```python
from build123d import *

# Parameters (mm, degrees)
SKETCH1_W           = 111
SKETCH1_H           = 170.0625
BOSS_EXTRUDE1_DEPTH = 3
SKETCH2_W           = 111
SKETCH2_H           = 170.0625
SKETCH2_W_2         = 105
SKETCH2_H_2         = 164.0625
BOSS_EXTRUDE2_DEPTH = 131.25
SKETCH3_R           = 47
CUT_EXTRUDE1_DEPTH  = 3


with BuildPart() as part:
    # Sketch1 → Boss-Extrude1 (new body)
    with BuildSketch(Plane(origin=(0, 0, 0), x_dir=(1, 0, 0), z_dir=(0, 1, 0))):
        with Locations((55.5, -85.03125)):
            Rectangle(SKETCH1_W, SKETCH1_H)
    extrude(amount=BOSS_EXTRUDE1_DEPTH)

    # Sketch2 → Boss-Extrude2 (add)
    with BuildSketch(Plane(origin=(0, 3, 0), x_dir=(1, 0, 0), z_dir=(0, 1, 0))):
        with Locations((55.5, -85.03125)):
            Rectangle(SKETCH2_W, SKETCH2_H)
        with Locations((55.5, -85.03125)):
            Rectangle(SKETCH2_W_2, SKETCH2_H_2, mode=Mode.SUBTRACT)
    extrude(amount=BOSS_EXTRUDE2_DEPTH)

    # Sketch3 → Cut-Extrude1 (cut)
    with BuildSketch(Plane(origin=(0, 0, 0), x_dir=(-1, 0, 0), z_dir=(0, -1, 0))):
        with Locations(Location((-55.5, -85.03125, 0), (0, 0, 90))):
            Circle(SKETCH3_R)
    extrude(amount=-CUT_EXTRUDE1_DEPTH, mode=Mode.SUBTRACT)


solid = part.part
```
Read the model definition and answer for the solid it produces. Units are mm, in the model's axes. A direction names the side the tool comes from. Round coordinates to 2 decimals unless told otherwise and drop trailing zeros. Write each loop counter-clockwise with the first axis right and the second up, starting at its lowest first coordinate (ties: lowest second). Pieces come first, ordered by that corner, then holes. Notation, with made-up numbers: (-11, 5) - (26, 5) arc R18 ccw to (26, 9) - close; hole circle Ø3 at (88, 39.5). An arc over 180 degrees is marked (long way). One line per item, written item: value.
Q1. For a pull along X with two mould halves and no side action, classify faces 3 (the flat face through (55, 68, 167.062)), 4 (the flat face through (111, 66, 86)), 5 (the flat face through (0, 66, 86)) as pulls with the +X half, pulls with the -X half, needs draft (parallel to the pull), parting line crosses it, or undercut.
The answers:
face 3: undercut
face 4: pulls with the +X half
face 5: pulls with the -X half
Q2. Straight lines are drawn through the part: line 1 (X direction, y = 58.5, z = 97.5); line 2 (Z direction, x = 15.5, y = 82); line 3 (Y direction, x = 76, z = 128). For each, find the intervals that lie inside material, in ascending order. Write a range as from..to.
The answers:
line 1: x = 0..3, 108..111
line 2: z = 0..3, 167.06..170.06
line 3: y = 0..3
Q3. Find section B-B (y = 40). Determine the outline of the cut face in (x, z), and give its area (3 significant figures).
The answers:
outline: (0, 0) - (111, 0) - (111, 170.06) - (0, 170.06) - close; hole (3, 3) - (108, 3) - (108, 167.06) - (3, 167.06) - close
area: 1,650 mm2
Q4. Find section C-C (z = 87). Determine the outline of the cut face in (x, y).
The answers:
outline: (0, 0) - (8.54, 0) - (8.54, 3) - (3, 3) - (3, 134.25) - (0, 134.25) - close; (102.46, 0) - (111, 0) - (111, 134.25) - (108, 134.25) - (108, 3) - (102.46, 3) - close
Q5. Which of the six approach directions +Z, -Z, +X, -X, +Y, -Y give full straight-line access (tool end or side, diameter ignored) to faces 1 (the flat face through (2, 134.25, 59)), 2 (the flat face through (8, 3, 84))?
The answers:
face 1: +Z, -Z, +X, -X, +Y
face 2: +Y
Q6. Find section D-D (z = 20.5). Determine the outline of the cut face in (x, y), and give its area (3 significant figures).
The answers:
outline: (0, 0) - (111, 0) - (111, 134.25) - (108, 134.25) - (108, 3) - (3, 3) - (3, 134.25) - (0, 134.25) - close
area: 1,120 mm2
Q7. This flat-tipped pin is pushed along its axis until it touches: P1, Ø10, axis at x = 29, z = 114, coming from the -Y side. Where does it stop, or does it pass through?
The answers:
P1: passes through
Q8. Find section A-A (x = 55.5). Determine the outline of the cut face in (y, z).
The answers:
outline: (0, 0) - (134.25, 0) - (134.25, 3) - (3, 3) - (3, 38.03) - (0, 38.03) - close; (0, 132.03) - (3, 132.03) - (3, 167.06) - (134.25, 167.06) - (134.25, 170.06) - (0, 170.06) - close
